Autodesk Inventor part; units mm, degrees
ref_plane "YZ Plane" through (0, 0, 0) normal (1, 0, 0) x (0, 1, 0)
ref_plane "XZ Plane" through (0, 0, 0) normal (0, 1, 0) x (-1, 0, 0)
ref_plane "XY Plane" through (0, 0, 0) normal (0, 0, 1) x (1, 0, 0)
sketch "Szkic1" plane through (0, 0, 0) normal (0, 0, 1) x (1, 0, 0)
  line L0 (0, 0) -> (45, 0) construction
  line L1 (45, 0) -> (45, 45) construction
  line L2 (45, 45) -> (0, 45) construction
  line L3 (0, 45) -> (0, 0) construction
  line L4 (0, 45) -> (22.5, 45) construction
  line L5 (45, 0) -> (45, 22.5) construction
  line L6 (22.5, 45) -> (0, 45)
  line L7 (0, 45) -> (0, 0)
  line L8 (0, 0) -> (45, 0)
  line L9 (45, 0) -> (45, 22.5)
  line L10 (22.5, 45) -> (22.5, 64)
  line L11 (45, 22.5) -> (64, 22.5)
  line L12 (22.5, 64) -> (32.5, 64)
  line L13 (64, 22.5) -> (64, 32.5)
  arc A0 (32.5, 64) -> (64, 32.5) centre (75.8985, 75.8985) ccw
  dimension "d0" = 45
  dimension "d1" = 45
  dimension "d2" = 22.5
  dimension "d3" = 19
  dimension "d4" = 19
  dimension "d5" = 10
  dimension "d6" = 10
  dimension "d7" = 45
extrude "Wyciągnięcie proste1" add sketch "Szkic1" along normal blind 6
equation "\"d0\" = d1"
equation "\"d3\" = d4"
equation "\"d5\" = d6"
properties part number "zamek_II_boki"
For this review, take the finished solid that the model builds, in its own axes (mm). A direction names the side the tool comes from. Round coordinates to 2 decimals unless told otherwise and drop trailing zeros. Loops run counter-clockwise (first coordinate to the right, second up) from the corner with the lowest first, then second, coordinate; pieces in that order, holes last.
(1) Clearance check with flat-ended pins moving along their axes: P1, Ø1.5, axis at x = 47, z = 4.5, coming from the -Y side; P2, Ø1.8, axis at y = 7, z = 2.5, coming from the +X side; P3, Ø1.5, axis at x = 39, z = 4, coming from the +Y side; P4, Ø3, axis at x = 47.5, y = 14.5, coming from the +Z side. State where each tip first meets the part, or that it passes through.
Returned:
P1: stops at y = 22.5
P2: stops at x = 45
P3: stops at y = 51.25
P4: passes through
(2) Wall thickness on line 1 along X through (y, z) = (4, 0.7); line 2 along X through (y, z) = (43.5, 3.7): over which ranges is each line inside the solid? List them lowest first.
Returned:
line 1: x = 0 to 45
line 2: x = 0 to 44.67
(3) We need section B-B (x = 10.5). Give the boundary of the cut face in (y, z).
Returned:
outline: (0, 0) - (45, 0) - (45, 6) - (0, 6) - close
(4) We need section A-A (z = 2.4). Give the boundary of the cut face in (x, y).
Returned:
outline: (0, 0) - (45, 0) - (45, 22.5) - (64, 22.5) - (64, 32.5) arc R45 cw to (32.5, 64) - (22.5, 64) - (22.5, 45) - (0, 45) - close
(5) Tool access review of faces 1 (the flat face through (45, 11, 3)), 2 (the flat face through (24, 25, 0)), 3 (the flat face through (22.5, 54, 3)): name each direction out of +Z, -Z, +X, -X, +Y, -Y from which nothing blocks a thin tool from reaching the whole face with its end or side.
Returned:
face 1: +Z, -Z, +X, -Y
face 2: -Z, +X, -X, +Y, -Y
face 3: +Z, -Z, -X, +Y
